Read the model definition and answer for the solid it produces. Units are mm, in the model's axes. Coordinates: 2 decimals unless noted, no trailing zeros. Write each loop counter-clockwise with the first axis right and the second up, starting at its lowest first coordinate (ties: lowest second). Pieces come first, ordered by that corner, then holes. Notation, with made-up numbers: (14.5, -19.75) -> (53.5, -19.75) arc R17 ccw to (53.5, -3.75) -> close; hole circle Ø1 at (-24.75, 68.25). An arc over 180 degrees is marked (long way). Use CSV: the item, a comma, the result in double quotes.
from build123d import *

# Parameters (mm, degrees)
SKETCH1_R           = 3.4925
BOSS_EXTRUDE1_DEPTH = 76.2


with BuildPart() as part:
    # Sketch1 → Boss-Extrude1 (new body, symmetric)
    with BuildSketch(Plane(origin=(0, 0, 0), x_dir=(0, 0, -1), z_dir=(1, 0, 0))):
        with BuildLine():
            Line((-25.4, -6.35), (25.4, -6.35))
            ThreePointArc((25.4, -6.35), (31.75, 0), (25.4, 6.35))
            Line((25.4, 6.35), (-25.4, 6.35))
            ThreePointArc((-25.4, 6.35), (-31.75, 0), (-25.4, -6.35))
        make_face()
        with Locations((-25.4, 0)):
            Circle(SKETCH1_R, mode=Mode.SUBTRACT)
        with Locations((25.4, 0)):
            Circle(SKETCH1_R, mode=Mode.SUBTRACT)
        Circle(SKETCH1_R, mode=Mode.SUBTRACT)
    extrude(amount=BOSS_EXTRUDE1_DEPTH, both=True)


solid = part.part
1. A cutting plane is placed at A-A (z = 0). Give the vertices of the cut face in (x, y).
Solutions:
outline,"(-76.2, -6.35) -> (76.2, -6.35) -> (76.2, -3.49) -> (-76.2, -3.49) -> close; (-76.2, 3.49) -> (76.2, 3.49) -> (76.2, 6.35) -> (-76.2, 6.35) -> close"
2. Each of these flat-tipped pins is pushed along its axis until it touches: pin 1 Ø1 at (x, y) = (55.5, -1.5) entering from +Z; pin 2 Ø4 at (x, y) = (-53, -4) entering from +Z. Where does it stop, or does it pass through?
Solutions:
pin 1,"stops at z = 31.67"
pin 2,"stops at z = 31.43"
3. A cutting plane is placed at C-C (x = 59). Give the number of separate pieces and of enclosed holes in the cut face, and give its area (3 significant figures).
Solutions:
separate pieces,"1"
enclosed holes,"3"
area,"657 mm^2"
4. A cutting plane is placed at B-B (y = 0). Give the vertices of the cut face in (x, z), and give its area (3 significant figures).
Solutions:
outline,"(-76.2, -31.75) -> (76.2, -31.75) -> (76.2, -28.89) -> (-76.2, -28.89) -> close; (-76.2, -21.91) -> (76.2, -21.91) -> (76.2, -3.49) -> (-76.2, -3.49) -> close; (-76.2, 3.49) -> (76.2, 3.49) -> (76.2, 21.91) -> (-76.2, 21.91) -> close; (-76.2, 28.89) -> (76.2, 28.89) -> (76.2, 31.75) -> (-76.2, 31.75) -> close"
area,"6,480 mm^2"
5. Find the intervals of material crossed by line 1 along Y through (x, z) = (34, 0); line 2 along Z through (x, y) = (29, 1.5); line 3 along Z through (x, y) = (-17, -0.75), in increasing order.
Solutions:
line 1,"y = -6.35 to -3.49, 3.49 to 6.35"
line 2,"z = -31.57 to -28.55, -22.25 to -3.15, 3.15 to 22.25, 28.55 to 31.57"
line 3,"z = -31.71 to -28.81, -21.99 to -3.41, 3.41 to 21.99, 28.81 to 31.71"
